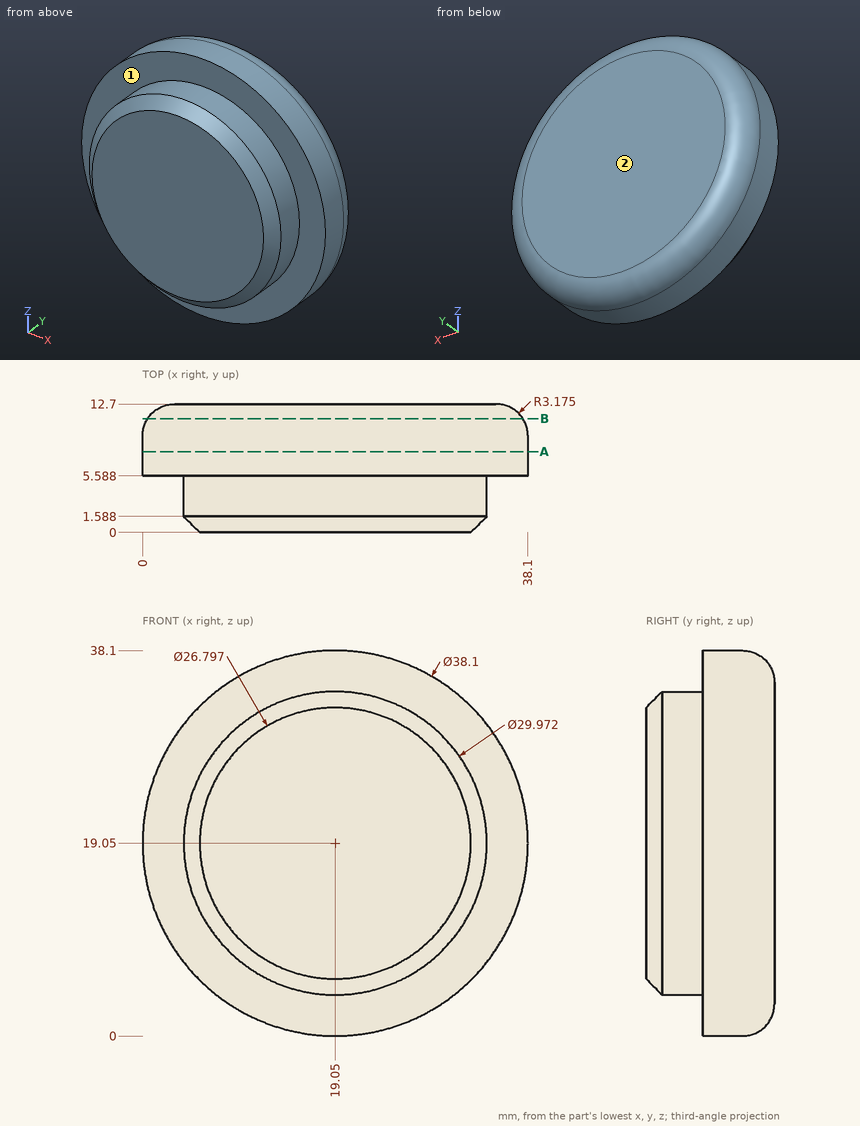
The drawing under review shows one solid part. Ordinate dimensions are in mm from its lowest x, y, z. A direction names the side the tool comes from. Round coordinates to 2 decimals unless told otherwise and drop trailing zeros. Order: outer loops, then holes, each group sorted by start corner. A loop starts at its lowest first (then second) coordinate and runs counter-clockwise, first axis right, second up. Notation, with made-up numbers: (-26, 17.25) -> (31, 17.25) arc R17 cw to (31, 27.25) -> close; hole circle Ø9 at (48.25, 8). An arc over 180 degrees is marked (long way). Return JSON: item names as keys, results as strings.
1. For the marked faces 1 and 2, list the 3-axis set-ups (+Z, -Z, +X, -X, +Y, -Y) from which the entire face can be reached by the end or side of a thin tool; tool diameter is ignored.
Answer block:
{"face 1": "-Y", "face 2": "+Z, -Z, +X, -X, +Y"}
2. Take a section at B-B (y = 11.25). Write out the cut boundary in (x, z).
Answer block:
{"outline": "circle Ø37.08 at (19.05, 19.05)"}
3. Insertion check: P1, Ø6, axis at x = 26.5, y = 11.5, coming from the +Z side (1 decimal); P2, Ø4, axis at y = 9.5, z = 30, coming from the -X side; P3, Ø4, axis at x = 16.5, y = 6, coming from the -Z side. Each pin has a flat end and moves straight along its axis. Give the tip position at first contact, or say it passes through.
Answer block:
{"P1": "stops at z = 37.4", "P2": "stops at x = 2.23", "P3": "stops at z = 0.01"}
4. Take a section at A-A (y = 8). Write out the cut boundary in (x, z), then the cut area to 3 significant figures.
Answer block:
{"outline": "circle Ø38.1 at (19.05, 19.05)", "area": "1,140 mm²"}
5. For L1, parallel to Z at x = 19, y = 5.75; L2, parallel to Y at x = 9.5, z = 31; L3, parallel to X at y = 9.75, z = 32.5, list the stretches that pass through material, from the lowest coordinate up. Write a range as [from, to].
Answer block:
{"L1": "z = [0, 38.1]", "L2": "y = [5.59, 12.7]", "L3": "x = [5.57, 32.53]"}
